The listing builds one solid part. Answer for the finished solid, in the listing's coordinates (mm). Face numbers are marked on the shaded views. Coordinates: 2 decimals unless noted, no trailing zeros.
```python
from build123d import *

# Parameters (mm, degrees)
EXTRUDE_1_DEPTH     = 4.5
CUT_EXTRUDE_1_DEPTH = 1
SKETCH_3_R          = 2.5
SKETCH_3_R_2        = 1.65
CUT_EXTRUDE_2_DEPTH = 3.4
EXTRUDE_2_DEPTH     = 8
EXTRUDE_2_TAPER     = 30


with BuildPart() as part:
    # 草图1 → 凸台-拉伸1 (new body)
    with BuildSketch(Plane(origin=(0, 0, 0), x_dir=(1, 0, 0), z_dir=(0, 1, 0))):
        with BuildLine():
            Line((-36, 21.5), (36, 21.5))
            ThreePointArc((36, 21.5), (40.242640687, 19.742640687), (42, 15.5))
            Line((42, 15.5), (42, -15.5))
            ThreePointArc((42, -15.5), (40.242640687, -19.742640687), (36, -21.5))
            Line((36, -21.5), (-36, -21.5))
            ThreePointArc((-36, -21.5), (-40.242640687, -19.742640687), (-42, -15.5))
            Line((-42, -15.5), (-42, 15.5))
            ThreePointArc((-42, 15.5), (-40.242640687, 19.742640687), (-36, 21.5))
        make_face()
    extrude(amount=EXTRUDE_1_DEPTH)

    # 草图2 → 切除-拉伸1 (cut)
    with BuildSketch(Plane.XZ):
        with BuildLine():
            Line((36, 20.5), (-36, 20.5))
            ThreePointArc((-36, 20.5), (-39.535533906, 19.035533906), (-41, 15.5))
            Line((-41, 15.5), (-41, -15.5))
            ThreePointArc((-41, -15.5), (-39.535533906, -19.035533906), (-36, -20.5))
            Line((-36, -20.5), (36, -20.5))
            ThreePointArc((36, -20.5), (39.535533906, -19.035533906), (41, -15.5))
            Line((41, -15.5), (41, 15.5))
            ThreePointArc((41, 15.5), (39.535533906, 19.035533906), (36, 20.5))
        make_face()
    extrude(amount=-CUT_EXTRUDE_1_DEPTH, mode=Mode.SUBTRACT)

    # 草图3 → 切除-拉伸2 (cut)
    # profile 1 of 5: a face of its own
    with BuildSketch(Plane(origin=(0, 1, 0), x_dir=(-1, 0, 0), z_dir=(0, -1, 0))):
        with BuildLine():
            Line((-41, 15.5), (-41, -15.5))
            ThreePointArc((-41, -15.5), (-39.535533906, -19.035533906), (-36, -20.5))
            Line((-36, -20.5), (36, -20.5))
            ThreePointArc((36, -20.5), (39.535533906, -19.035533906), (41, -15.5))
            Line((41, -15.5), (41, 15.5))
            ThreePointArc((41, 15.5), (39.535533906, 19.035533906), (36, 20.5))
            Line((36, 20.5), (-36, 20.5))
            ThreePointArc((-36, 20.5), (-39.535533906, 19.035533906), (-41, 15.5))
        make_face()
        with Locations(Location((36, 15.5, 0), (0, 0, 90))):
            Circle(SKETCH_3_R, mode=Mode.SUBTRACT)
        with Locations(Location((36, -15.5, 0), (0, 0, 90))):
            Circle(SKETCH_3_R, mode=Mode.SUBTRACT)
        with Locations(Location((-36, 15.5, 0), (0, 0, 90))):
            Circle(SKETCH_3_R, mode=Mode.SUBTRACT)
        with Locations(Location((-36, -15.5, 0), (0, 0, 90))):
            Circle(SKETCH_3_R, mode=Mode.SUBTRACT)
    # profile 2 of 5: a face of its own
    with BuildSketch(Plane(origin=(0, 1, 0), x_dir=(-1, 0, 0), z_dir=(0, -1, 0))):
        with Locations(Location((36, 15.5, 0), (0, 0, 90))):
            Circle(SKETCH_3_R_2)
    # profile 3 of 5: a face of its own
    with BuildSketch(Plane(origin=(0, 1, 0), x_dir=(-1, 0, 0), z_dir=(0, -1, 0))):
        with Locations(Location((36, -15.5, 0), (0, 0, 90))):
            Circle(SKETCH_3_R_2)
    # profile 4 of 5: a face of its own
    with BuildSketch(Plane(origin=(0, 1, 0), x_dir=(-1, 0, 0), z_dir=(0, -1, 0))):
        with Locations(Location((-36, -15.5, 0), (0, 0, 90))):
            Circle(SKETCH_3_R_2)
    # profile 5 of 5: a face of its own
    with BuildSketch(Plane(origin=(0, 1, 0), x_dir=(-1, 0, 0), z_dir=(0, -1, 0))):
        with Locations(Location((-36, 15.5, 0), (0, 0, 90))):
            Circle(SKETCH_3_R_2)
    extrude(amount=-CUT_EXTRUDE_2_DEPTH, mode=Mode.SUBTRACT)

    # 草图5 → 凸台-拉伸2 (add)
    with BuildSketch(Plane(origin=(0, 4.5, 0), x_dir=(1, 0, 0), z_dir=(0, 1, 0))):
        with BuildLine():
            Line((42, -15.5), (42, 15.5))
            ThreePointArc((42, 15.5), (40.242640687, 19.742640687), (36, 21.5))
            Line((36, 21.5), (-36, 21.5))
            ThreePointArc((-36, 21.5), (-40.242640687, 19.742640687), (-42, 15.5))
            Line((-42, 15.5), (-42, -15.5))
            ThreePointArc((-42, -15.5), (-40.242640687, -19.742640687), (-36, -21.5))
            Line((-36, -21.5), (36, -21.5))
            ThreePointArc((36, -21.5), (40.242640687, -19.742640687), (42, -15.5))
        make_face()
    extrude(amount=EXTRUDE_2_DEPTH, taper=EXTRUDE_2_TAPER)


solid = part.part
```
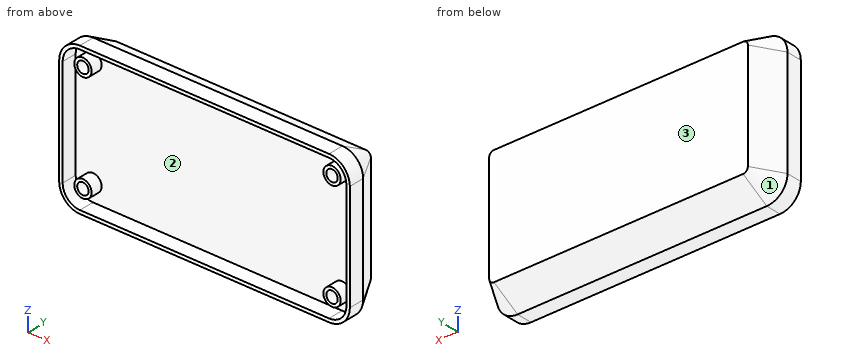
(1) Consider line 1 (X direction, y = 3.2, z = -15.5); line 2 (X direction, y = 1.5, z = 17); line 3 (Y direction, x = -20, z = 12). Determine where each line is inside the solid, lowest interval first.
(2) Each of these flat-tipped pins is pushed along its axis until it touches: pin 1 Ø1.5 at (x, z) = (-36.5, -15) entering from -Y; pin 2 Ø3.5 at (x, z) = (35.5, 14.5) entering from -Y; pin 3 Ø1.5 at (x, y) = (16, 7) entering from +Z. Where does it stop, or does it pass through?
(3) The mould has two halves that part along Z. Classify the marked faces 1, 2 and 3: released by +Z, released by -Z, zero draft, split by the parting line, or undercut.
(4) Find section A-A (y = 3). Give the number of separate pieces and of enclosed holes in the cut face, and give its area (3 significant figures).
Findings below:
1. line 1: x = -42 to -41, -38.5 to -37.65, -34.35 to -33.5, 33.5 to 34.35, 37.65 to 38.5, 41 to 42
1. line 2: x = -41.81 to -40.77, -38 to -36.69, -35.31 to -34, 34 to 35.31, 36.69 to 38, 40.77 to 41.81
1. line 3: y = 4.4 to 12.5
2. pin 1: stops at y = 4.4
2. pin 2: stops at y = 1
2. pin 3: stops at z = 20.49
3. face 1: released by -Z
3. face 2: undercut
3. face 3: zero draft
4. separate pieces: 5
4. enclosed holes: 5
4. area: 285 mm2
